from build123d import *

# Parameters (mm, degrees)
CHAMFER1_SIZE = 0.25
HEX_2_DEPTH   = 2.4


with BuildPart() as part:
    # BodySke → BaseBody (revolve)
    with BuildSketch(Plane.XY, mode=Mode.PRIVATE) as basebody_sk:
        with BuildLine():
            Line((0, 0), (0, 5))
            Line((0, 5), (4.5, 5))
            Line((4.5, 5), (4.5, 2.96))
            ThreePointArc((4.5, 2.96), (4.573223305, 2.783223305), (4.75, 2.71))
            Line((4.75, 2.71), (6.715, 2.71))
            Line((6.715, 2.71), (7, 2.995))
            Line((7, 2.995), (34.5, 2.995))
            Line((34.5, 2.995), (34.5, 2.34))
            ThreePointArc((34.5, 2.34), (34.646446609, 1.986446609), (35, 1.84))
            Line((35, 1.84), (36.5, 1.84))
            Line((36.5, 1.84), (37.16, 2.5))
            Line((37.16, 2.5), (43.805, 2.5))
            Line((43.805, 2.5), (44.25, 2.055))
            Line((44.25, 2.055), (44.25, 0))
            Line((44.25, 0), (0, 0))
        make_face()
    revolve(basebody_sk.sketch.rotate(Axis((-6.35, 0, 0), (1, 0, 0)), 90), axis=Axis((-6.35, 0, 0), (1, 0, 0)))

    # Chamfer1
    chamfer1_edges = [part.edges().sort_by_distance(p)[0] for p in [
        (0, 0, -5),
    ]]
    chamfer(chamfer1_edges, length=CHAMFER1_SIZE)

    # Sketch2 → PreBroach (revolve, cut)
    with BuildSketch(Plane.XY, mode=Mode.PRIVATE) as prebroach_sk:
        Polygon((0, 1.54), (2.4, 1.54), (3.289119415, 0), (0, 0), align=None)
    revolve(prebroach_sk.sketch.rotate(Axis((0, 0, 0), (1, 0, 0)), 90), axis=Axis((0, 0, 0), (1, 0, 0)), mode=Mode.SUBTRACT)

    # Sketch3 → Hex 2 (cut)
    with BuildSketch(Plane.ZY):
        Polygon((-1.54, -0.889119415), (-1.54, 0.889119415), (0, 1.778238829), (1.54, 0.889119415), (1.54, -0.889119415), (0, -1.778238829), align=None)
    extrude(amount=-HEX_2_DEPTH, mode=Mode.SUBTRACT)


solid = part.part
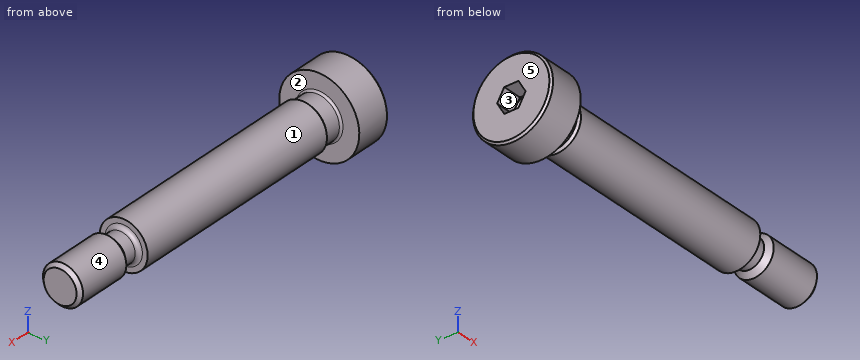
Read the model definition and answer for the solid it produces. Units are mm, in the model's axes. Face numbers are marked on the shaded views. A direction names the side the tool comes from. Coordinates: 2 decimals unless noted, no trailing zeros. Write each loop counter-clockwise with the first axis right and the second up, starting at its lowest first coordinate (ties: lowest second). Pieces come first, ordered by that corner, then holes. Notation, with made-up numbers: (11, -29.5) -> (46, -29.5) arc R33 cw to (46, 0.5) -> close; hole circle Ø1 at (81, 20). An arc over 180 degrees is marked (long way). Return JSON: item names as keys, results as strings.
(1) Each of these flat-tipped pins is pushed along its axis until it touches: P1, Ø0.6, axis at y = 1, z = -1, coming from the -X side; P2, Ø1.5, axis at x = 39, y = -2, coming from the +Z side; P3, Ø4, axis at x = 37, y = 4, coming from the -Z side; P4, Ø4, axis at x = 31.5, z = -0.5, coming from the -Y side (3 decimals). Where does it stop, or does it pass through?
Answers below:
{"P1": "x = 0", "P2": "z = 2.17", "P3": "z = -1.49", "P4": "y = -2.995"}
(2) For a pull along Y with two mould halves and no side action, classify the marked faces 1, 2 and 3 as pulls with the +Y half, pulls with the -Y half, needs draft (parallel to the pull), parting line crosses it, or undercut.
Answers below:
{"face 1": "parting line crosses it", "face 2": "needs draft", "face 3": "undercut"}
(3) Which of the six approach directions +Z, -Z, +X, -X, +Y, -Y give full straight-line access (tool end or side, diameter ignored) to the marked faces 4 and 5?
Answers below:
{"face 4": "+X", "face 5": "+Z, -Z, -X, +Y, -Y"}
(4) Consider line 1 along X through (y, z) = (2, 2.5); line 2 along X through (y, z) = (2.25, 0.5); line 3 along X through (y, z) = (0.25, 2). Determine where each line is inside the solid, lowest interval first. Write a range as from..to.
Answers below:
{"line 1": "0..4.5", "line 2": "0..34.5, 36.96..44", "line 3": "0..34.62, 36.68..44.25"}
(5) The part is cut by section A-A on x = 26. Give the vertices of the cut face in (y, z) (3 decimals).
Answers below:
{"outline": "circle Ø5.99 at (0, 0)"}
